Geometry: final body of the model. Coordinates: model frame, mm. A direction names the side the tool comes from. Give positions to 0.01 mm unless a question says otherwise; leave off trailing zeros. Order: outer loops, then holes, each group sorted by start corner. A loop starts at its lowest first (then second) coordinate and runs counter-clockwise, first axis right, second up. Notation, with made-up numbers: (16, 77.5) -> (61, 77.5) arc R31 cw to (61, 115.5) -> close; hole circle Ø1 at (61.25, -8.75). An arc over 180 degrees is marked (long way). One line per question, with ' | ' between items. Start each with the question number.
(1) Section C-C (x = 6). Return loops of the section in (y, z), then the cut area to 3 significant figures.
(2) Ray query, L1, parallel to Y at x = 11, z = -0.75 (3 decimals); L2, parallel to Z at x = 8.25, y = 5.5; L3, parallel to X at y = 9.3, z = -7.5. Return the intervals inside material, ascending.
(3) Set-up query: faces 1 (the face through (11.808, 14.364, -0.862)), 2 (the face through (13, 14, -1.7)), 3 (the face through (11, 6, -10.5)). Return all of +Z, -Z, +X, -X, +Y, -Y with unobstructed straight access to the full face (end or side cutting, diameter ignored); none if empty.
(4) Section A-A (y = 18). Return loops of the section in (x, z) (3 decimals).
(5) Section B-B (z = -27.3). Return loops of the section in (x, y), then the cut area to 3 significant figures.
(6) Mould query, pull axis Z, two halves, no side actions, for faces 4 (the face through (11, 8, -8)), 5 (the face through (21, 24, -1)), 6 (the face through (1.141, 5.324, -38.797)). Classes: +Z half, -Z half, draft (parallel to the pull), parting line (faces both ways), or undercut.
(7) Section D-D (z = -15). Return loops of the section in (x, y).
(8) First-contact query: pin 1 Ø1.1 at (x, z) = (11, -35.5) entering from +Y; pin 2 Ø1.1 at (x, z) = (10.5, -7) entering from +Y; pin 3 Ø12 at (x, y) = (2.5, 18.5) entering from -Z. Flat tips, straight axial feed; report the tip coordinate or a pass-through.
```python
from build123d import *

# Parameters (mm, degrees)
SKETCH1_W           = 22
SKETCH1_H           = 40
BOSS_EXTRUDE1_DEPTH = 10.5
SKETCH2_W           = 13
SKETCH2_H           = 23
CUT_EXTRUDE1_DEPTH  = 8.5
SKETCH3_R           = 5.85
CUT_EXTRUDE2_DEPTH  = 47.435439053
SKETCH4_W           = 22
SKETCH4_H           = 1.7
BOSS_EXTRUDE2_DEPTH = 14
SKETCH5_R           = 3.725
CUT_EXTRUDE3_DEPTH  = 51.508811113
SKETCH5_3_R         = 3.725
SKETCH5_3_R_2       = 0.7
CUT_EXTRUDE4_DEPTH  = 10
SKETCH6_R           = 0.7
CUT_EXTRUDE5_DEPTH  = 2.5
FILLET1_R           = 4
FILLET2_R           = 2.5
CUT_EXTRUDE6_DEPTH  = 10


with BuildPart() as part:
    # Sketch1 → Boss-Extrude1 (new body)
    with BuildSketch(Plane(origin=(0, 0, 0), x_dir=(1, 0, 0), z_dir=(0, 1, 0))):
        with Locations((11, 20)):
            Rectangle(SKETCH1_W, SKETCH1_H)
    extrude(amount=BOSS_EXTRUDE1_DEPTH)

    # Sketch2 → Cut-Extrude1 (cut)
    with BuildSketch(Plane(origin=(0, 10.5, 0), x_dir=(1, 0, 0), z_dir=(0, 1, 0))):
        with Locations((11, 22)):
            Rectangle(SKETCH2_W, SKETCH2_H)
    extrude(amount=-CUT_EXTRUDE1_DEPTH, mode=Mode.SUBTRACT)

    # Sketch3 → Cut-Extrude2 (cut, through all)
    with BuildSketch(Plane(origin=(0, 2, 0), x_dir=(1, 0, 0), z_dir=(0, 1, 0))):
        with Locations(Location((11, 27.3, 0), (0, 0, 270))):
            Circle(SKETCH3_R)
    extrude(amount=-CUT_EXTRUDE2_DEPTH, mode=Mode.SUBTRACT)

    # Sketch4 → Boss-Extrude2 (add)
    with BuildSketch(Plane(origin=(0, 10.5, 0), x_dir=(1, 0, 0), z_dir=(0, 1, 0))):
        with Locations((11, 0.85)):
            Rectangle(SKETCH4_W, SKETCH4_H)
    extrude(amount=BOSS_EXTRUDE2_DEPTH)

    # Sketch5 → Cut-Extrude3 (cut, through all)
    with BuildSketch(Plane(origin=(0, 0, -1.7), x_dir=(-1, 0, 0), z_dir=(0, 0, -1))):
        with Locations((-11, 18)):
            Circle(SKETCH5_R)
    extrude(amount=-CUT_EXTRUDE3_DEPTH, mode=Mode.SUBTRACT)

    # Sketch5_3 → Cut-Extrude4 (cut)
    with BuildSketch(Plane(origin=(0, 0, -1.7), x_dir=(-1, 0, 0), z_dir=(0, 0, -1))):
        with Locations((-11, 18)):
            Circle(SKETCH5_3_R)
        with Locations((-17.725, 18)):
            Circle(SKETCH5_3_R_2)
        with Locations((-4.275, 18)):
            Circle(SKETCH5_3_R_2)
    extrude(amount=-CUT_EXTRUDE4_DEPTH, mode=Mode.SUBTRACT)

    # Sketch6 → Cut-Extrude5 (cut)
    with BuildSketch(Plane(origin=(0, 10.5, 0), x_dir=(1, 0, 0), z_dir=(0, 1, 0))):
        with Locations(Location((11, 35.5, 0), (0, 0, 270))):
            Circle(SKETCH6_R)
        with Locations(Location((11, 7.5, 0), (0, 0, 270))):
            Circle(SKETCH6_R)
    extrude(amount=-CUT_EXTRUDE5_DEPTH, mode=Mode.SUBTRACT)

    # Fillet1
    fillet1_edges = [part.edges().sort_by_distance(p)[0] for p in [
        (0, 5.25, -40),
        (22, 5.25, -40),
    ]]
    fillet(fillet1_edges, radius=FILLET1_R)

    # Fillet2
    fillet2_edges = [part.edges().sort_by_distance(p)[0] for p in [
        (0, 24.5, -0.85),
        (22, 24.5, -0.85),
    ]]
    fillet(fillet2_edges, radius=FILLET2_R)

    # Sketch7 → Cut-Extrude6 (cut)
    with BuildSketch(Plane(origin=(0, 2, 0), x_dir=(1, 0, 0), z_dir=(0, 1, 0))):
        with BuildLine():
            ThreePointArc((9.023699499, 21.833388834), (10.872986109, 18.699861887), (12.803373856, 21.784088734))
            ThreePointArc((12.803373856, 21.784088734), (10.909436036, 21.494356303), (9.023699499, 21.833388834))
        make_face()
    extrude(amount=-CUT_EXTRUDE6_DEPTH, mode=Mode.SUBTRACT)


solid = part.part
```
Response:
1) outline: (0, -40) -> (10.5, -40) -> (10.5, -33.5) -> (2, -33.5) -> (2, -30.34) -> (0, -30.34) -> close; (0, -24.26) -> (2, -24.26) -> (2, -10.5) -> (10.5, -10.5) -> (10.5, -1.7) -> (24.5, -1.7) -> (24.5, 0) -> (0, 0) -> close | area: 236 mm^2
2) L1: y = 0 to 14.275, 21.725 to 24.5 | L2: z = -40 to -33.5, -10.5 to 0 | L3: x = 0 to 10.3, 11.7 to 22
3) face 1: +Z, -Z | face 2: -Z, +X, -X, +Y | face 3: +Y
4) outline: (0, -1.7) -> (3.575, -1.7) -> (3.575, 0) -> (0, 0) -> close; (4.975, -1.7) -> (7.275, -1.7) -> (7.275, 0) -> (4.975, 0) -> close; (14.725, -1.7) -> (17.025, -1.7) -> (17.025, 0) -> (14.725, 0) -> close; (18.425, -1.7) -> (22, -1.7) -> (22, 0) -> (18.425, 0) -> close
5) outline: (0, 0) -> (5.15, 0) -> (5.15, 2) -> (4.5, 2) -> (4.5, 10.5) -> (0, 10.5) -> close; (16.85, 0) -> (22, 0) -> (22, 10.5) -> (17.5, 10.5) -> (17.5, 2) -> (16.85, 2) -> close | area: 97.1 mm^2
6) face 4: undercut | face 5: draft | face 6: -Z half
7) outline: (0, 0) -> (22, 0) -> (22, 10.5) -> (17.5, 10.5) -> (17.5, 2) -> (4.5, 2) -> (4.5, 10.5) -> (0, 10.5) -> close
8) pin 1: stops at y = 8 | pin 2: stops at y = 10.5 | pin 3: stops at z = -1.7
